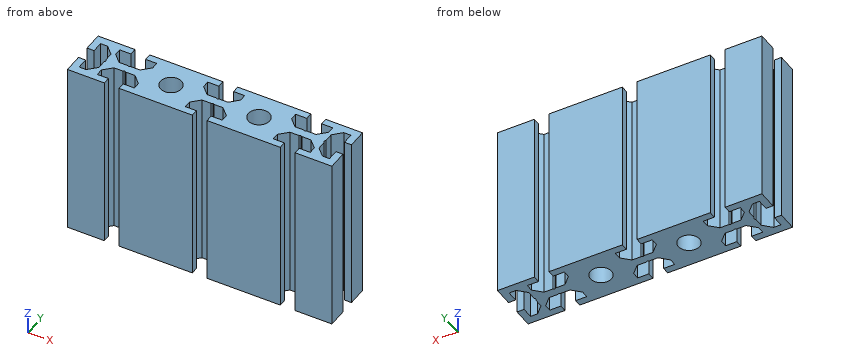
from build123d import *

# Parameters (mm, degrees)
SKETCH_1_R      = 6
EXTRUDE_1_DEPTH = 100


with BuildPart() as part:
    # 草图1 → 凸台-拉伸1 (new body)
    with BuildSketch(Plane.XY):
        Polygon((99.95, 4.2), (99.95, 15), (79.05, 15), (79.05, 11), (85.35, 11), (85.35, 7), (80.8, 2.45), (75.716025404, 2.45), (74.85, 1.95), (73.983974596, 2.45), (68.9, 2.45), (64.35, 7), (64.35, 11), (70.65, 11), (70.65, 15), (29.15, 15), (29.15, 11), (35.45, 11), (35.45, 7), (30.9, 2.45), (25.816025404, 2.45), (24.95, 1.95), (24.083974596, 2.45), (19, 2.45), (14.45, 7), (14.45, 11), (20.75, 11), (20.75, 15), (-20.75, 15), (-20.75, 11), (-14.45, 11), (-14.45, 7), (-19, 2.45), (-24.083974596, 2.45), (-24.95, 1.95), (-25.816025404, 2.45), (-30.9, 2.45), (-35.45, 7), (-35.45, 11), (-29.15, 11), (-29.15, 15), (-50.05, 15), (-50.05, 4.2), (-46.05, 4.2), (-46.05, 10.5), (-42.05, 10.5), (-37.5, 5.95), (-37.5, 0.866025404), (-37, 0), (-37.5, -0.866025404), (-37.5, -5.95), (-42.05, -10.5), (-46.05, -10.5), (-46.05, -4.2), (-50.05, -4.2), (-50.05, -15), (-29.15, -15), (-29.15, -11), (-35.45, -11), (-35.45, -7), (-30.9, -2.45), (-25.816025404, -2.45), (-24.95, -1.95), (-24.083974596, -2.45), (-19, -2.45), (-14.45, -7), (-14.45, -11), (-20.75, -11), (-20.75, -15), (20.75, -15), (20.75, -11), (14.45, -11), (14.45, -7), (19, -2.45), (24.083974596, -2.45), (24.95, -1.95), (25.816025404, -2.45), (30.9, -2.45), (35.45, -7), (35.45, -11), (29.15, -11), (29.15, -15), (70.65, -15), (70.65, -11), (64.35, -11), (64.35, -7), (68.9, -2.45), (73.983974596, -2.45), (74.85, -1.95), (75.716025404, -2.45), (80.8, -2.45), (85.35, -7), (85.35, -11), (79.05, -11), (79.05, -15), (99.95, -15), (99.95, -4.2), (95.95, -4.2), (95.95, -10.5), (91.95, -10.5), (87.4, -5.95), (87.4, -0.866025404), (86.9, 0), (87.4, 0.866025404), (87.4, 5.95), (91.95, 10.5), (95.95, 10.5), (95.95, 4.2), align=None)
        Circle(SKETCH_1_R, mode=Mode.SUBTRACT)
        with Locations((49.9, 0)):
            Circle(SKETCH_1_R, mode=Mode.SUBTRACT)
    extrude(amount=EXTRUDE_1_DEPTH)


solid = part.part
Can you work these out from the model? Positions are in its coordinate system, mm. Round coordinates to 2 decimals unless told otherwise and drop trailing zeros. Write each loop counter-clockwise with the first axis right and the second up, starting at its lowest first coordinate (ties: lowest second). Pieces come first, ordered by that corner, then holes. Notation, with made-up numbers: (68.25, 78.5) -> (99.25, 78.5) arc R18 ccw to (99.25, 88.5) -> close; hole circle Ø5 at (7, 69). An arc over 180 degrees is marked (long way). Use one line per item in the form item = value. Start each with the question number.
Q1. If I drill on probe 1 along X at (y, z) = (11.5, 25); probe 2 along Y at (x, z) = (20, 93); probe 3 along X at (y, z) = (7.5, 30), over which ranges is the centre line in solid material (lowest first)? Write a range as [from, to].
Q2. Imagine slicing it at C-C (z = 49.5). Count the separate pieces of the cut face and the enclosed holes in it, then the cut area to 3 significant figures.
Q3. Imagine slicing it at A-A (x = 49.9). Please give me the cut outline in (y, z), then the cut area to 3 significant figures.
Q4. Imagine slicing it at B-B (y = -8.5). Please give me the cut outline in (x, z).
Worked out:
q1.probe_1 = [-50.05, -29.15], [-20.75, 20.75], [29.15, 70.65], [79.05, 99.95]
q1.probe_2 = [-15, -11], [-2.45, 2.45], [11, 15]
q1.probe_3 = [-50.05, -46.05], [-39.05, -35.45], [-14.45, 14.45], [35.45, 64.35], [85.35, 88.95], [95.95, 99.95]
q2.separate_pieces = 1
q2.enclosed_holes = 2
q2.area = 2,730 mm^2
q3.outline = (-15, 0) -> (-6, 0) -> (-6, 100) -> (-15, 100) -> close; (6, 0) -> (15, 0) -> (15, 100) -> (6, 100) -> close
q3.area = 1,800 mm^2
q4.outline = (-50.05, 0) -> (-46.05, 0) -> (-46.05, 100) -> (-50.05, 100) -> close; (-40.05, 0) -> (-35.45, 0) -> (-35.45, 100) -> (-40.05, 100) -> close; (-14.45, 0) -> (14.45, 0) -> (14.45, 100) -> (-14.45, 100) -> close; (35.45, 0) -> (64.35, 0) -> (64.35, 100) -> (35.45, 100) -> close; (85.35, 0) -> (89.95, 0) -> (89.95, 100) -> (85.35, 100) -> close; (95.95, 0) -> (99.95, 0) -> (99.95, 100) -> (95.95, 100) -> close
